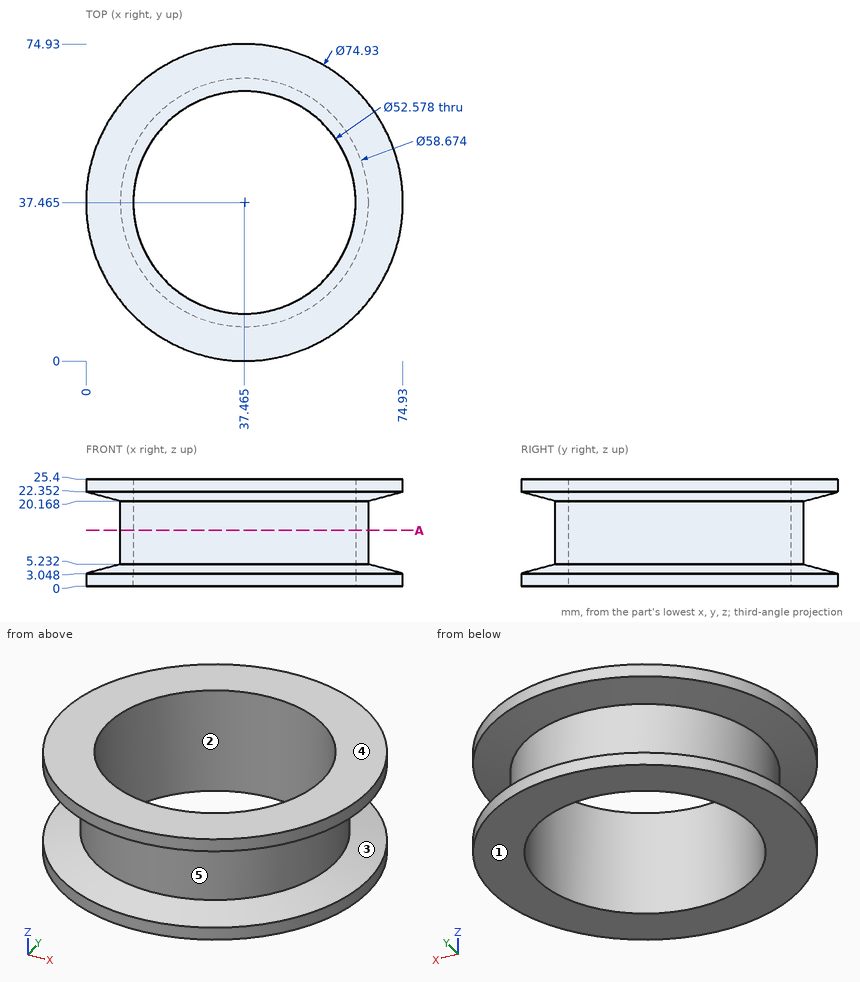
The drawing under review shows one solid part. Ordinate dimensions are in mm from its lowest x, y, z. A direction names the side the tool comes from. Give positions to 0.01 mm unless a question says otherwise; leave off trailing zeros. Write each loop counter-clockwise with the first axis right and the second up, starting at its lowest first coordinate (ties: lowest second). Pieces come first, ordered by that corner, then holes.
1. Draft analysis for pull direction X (two halves, no side actions). For the marked faces 1, 2 and 3, state which applies: +X half, -X half, draft (parallel to the pull), parting line (faces both ways), or undercut.
2. Tool access review of the marked faces 4 and 5: name each direction out of +Z, -Z, +X, -X, +Y, -Y from which nothing blocks a thin tool from reaching the whole face with its end or side.
3. Wall thickness on L1, parallel to X at y = 37, z = 16; L2, parallel to Z at x = 64.5, y = 15; L3, parallel to Y at x = 15, z = 14.5 (1 decimal): over which ranges is each line inside the solid? List them lowest first.
4. Add section A-A, the plane z = 13.25. Write out the cut boundary in (x, y) (1 decimal).
5. For P1, Ø3, axis at y = 41, z = 7, coming from the +X side; P2, Ø4, axis at x = 9, z = 13, coming from the -Y side (1 decimal); P3, Ø6, axis at x = 39, z = 17, coming from the -Y side, all flat-tipped, find the tip position at first contact; note any pin that passes through.
Worked answers:
1. face 1: draft
1. face 2: undercut
1. face 3: parting line
2. face 4: +Z, +X, -X, +Y, -Y
2. face 5: none
3. L1: x = 8.13 to 11.18, 63.75 to 66.8
3. L2: z = 0 to 3.67, 21.73 to 25.4
3. L3: y = 18.6 to 23.8, 51.1 to 56.3
4. outline: circle Ø58.7 at (37.5, 37.5); hole circle Ø52.6 at (37.5, 37.5)
5. P1: stops at x = 66.73
5. P2: stops at y = 24.8
5. P3: stops at y = 8.13
